CAD build for the part. Positions are in the model's coordinates, mm. Give positions to 0.01 mm unless a question says otherwise; leave off trailing zeros. Write each loop counter-clockwise with the first axis right and the second up, starting at its lowest first coordinate (ties: lowest second). Pieces come first, ordered by that corner, then holes. Notation, with made-up numbers: (60.25, -6) - (114.25, -6) arc R9 ccw to (114.25, 7) - close; hole circle Ø2 at (82, 60.5). An arc over 180 degrees is marked (long way). Put each result on its own line as item: value. Start each with the question number.
1. Mould opens along Y. For faces 1 (the cylindrical face through (-55.64, 105.96, 5.07)), 2 (the flat face through (76.5, 111.73, 4.93)), 3 (the cylindrical face through (56.503, 20.154, 4.93)) say: +Y half, -Y half, draft (parallel to the pull), parting line (faces both ways), or undercut.
2. Cut at C-C on x = 140. List the corners of the cut face in (y, z).
3. Wall check: line 1 (X direction, y = 20, z = 3); line 2 (X direction, y = 17.5, z = 8.5); line 3 (Y direction, x = 182.5, z = 9.25). Give the ranges that are in metal, low to high.
4. Cut at D-D on x = 100. List the corners of the cut face in (y, z), and give its area (3 significant figures).
5. Cut at B-B on y = 20. List the corners of the cut face in (x, z).
6. Cut at A-A on z = 3. Give the number of separate pieces and of enclosed holes in the cut face, and give its area (3 significant figures).
7. Drop flat-ended pins along their axis: pin 1 (5 mm diameter, centred on y = 101, z = 3, fed in from -X); pin 2 (4 mm diameter, centred on y = 56, z = 2.5, fed in from -X). Give the stop position or say it passes through.
from build123d import *

# Parameters (mm, degrees)
BOSS_EXTRU_1_DEPTH           = 10
CONG_1_R                     = 10
ENL_V_MAT_EXTRU_1_DEPTH      = 246.669614874
ENL_V_MAT_EXTRU_1_DEPTH_BACK = 246.669614874
ESQUISSE2_R                  = 3.5


with BuildPart() as part:
    # Esquisse1 → Boss.-Extru.1 (new body)
    with BuildSketch(Plane.XY):
        Polygon((0, 0), (-56.389768432, 105.925417234), (-46.037006628, 144.562450286), (200, 78.637033052), (200, 0), align=None)
    extrude(amount=BOSS_EXTRU_1_DEPTH)

    # Congé1
    cong_1_edges = [part.edges().sort_by_distance(p)[0] for p in [
        (0, 0, 5),
        (-56.389768432, 105.925417234, 5),
        (-46.037006628, 144.562450286, 5),
        (200, 78.637033052, 5),
        (200, 0, 5),
    ]]
    fillet(cong_1_edges, radius=CONG_1_R)

    # Esquisse2 → Enlèv. mat.-Extru.1 (cut, two sides: drawn at the far end of the back side and taken through both)
    with BuildSketch(Plane.XY.offset(10).offset(-ENL_V_MAT_EXTRU_1_DEPTH_BACK)):
        with Locations((-22.199276394, 117.469626112)):
            Circle(ESQUISSE2_R)
        with Locations((16.437756658, 107.116864308)):
            Circle(ESQUISSE2_R)
        with Locations((55.074789709, 96.764102504)):
            Circle(ESQUISSE2_R)
        with Locations((93.711822761, 86.4113407)):
            Circle(ESQUISSE2_R)
        with Locations((132.348855812, 76.058578895)):
            Circle(ESQUISSE2_R)
        with Locations((170.985888864, 65.705817091)):
            Circle(ESQUISSE2_R)
        with Locations((20, 20)):
            Circle(ESQUISSE2_R)
        with Locations((60, 20)):
            Circle(ESQUISSE2_R)
        with Locations((100, 20)):
            Circle(ESQUISSE2_R)
        with Locations((180, 20)):
            Circle(ESQUISSE2_R)
        with Locations((140, 20)):
            Circle(ESQUISSE2_R)
    extrude(amount=ENL_V_MAT_EXTRU_1_DEPTH + ENL_V_MAT_EXTRU_1_DEPTH_BACK, mode=Mode.SUBTRACT)


solid = part.part
Report:
1. face 1: parting line
1. face 2: +Y half
1. face 3: undercut
2. outline: (0, 0) - (16.5, 0) - (16.5, 10) - (0, 10) - close; (23.5, 0) - (94.71, 0) - (94.71, 10) - (23.5, 10) - close
3. line 1: x = -10.65 to 16.5, 23.5 to 56.5, 63.5 to 96.5, 103.5 to 136.5, 143.5 to 176.5, 183.5 to 200
3. line 2: x = -9.32 to 17.55, 22.45 to 57.55, 62.45 to 97.55, 102.45 to 137.55, 142.45 to 177.55, 182.45 to 200
3. line 3: y = 0 to 17.55, 22.45 to 83.33
4. outline: (0, 0) - (16.5, 0) - (16.5, 10) - (0, 10) - close; (23.5, 0) - (105.43, 0) - (105.43, 10) - (23.5, 10) - close
4. area: 984 mm²
5. outline: (-10.65, 0) - (16.5, 0) - (16.5, 10) - (-10.65, 10) - close; (23.5, 0) - (56.5, 0) - (56.5, 10) - (23.5, 10) - close; (63.5, 0) - (96.5, 0) - (96.5, 10) - (63.5, 10) - close; (103.5, 0) - (136.5, 0) - (136.5, 10) - (103.5, 10) - close; (143.5, 0) - (176.5, 0) - (176.5, 10) - (143.5, 10) - close; (183.5, 0) - (200, 0) - (200, 10) - (183.5, 10) - close
6. separate pieces: 1
6. enclosed holes: 11
6. area: 25,300 mm²
7. pin 1: stops at x = -55.02
7. pin 2: stops at x = -30.88
